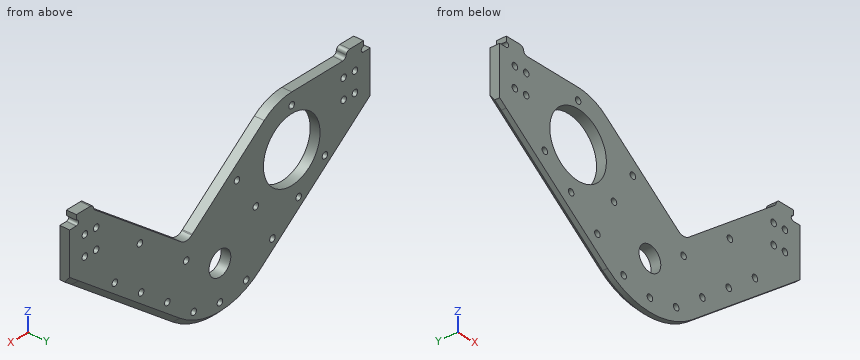
from build123d import *

# Parameters (mm, degrees)
SKETCH3_R                          = 17.8
SKETCH3_R_2                        = 7.9375
BOSS_EXTRUDE1_DEPTH                = 6.35
SKETCH7_R                          = 20.6375
CUT_EXTRUDE1_DEPTH                 = 7.35
SKETCH8_W                          = 4.7498
SKETCH8_H                          = 41.275
BOSS_EXTRUDE4_DEPTH                = 6.35
SKETCH10_R                         = 2.0193
SPACER_HOLES_DEPTH                 = 7.35
SPACER_HOLE_PATTERN_COUNT          = 5
SPACER_HOLE_PATTERN_PITCH          = 24.13
SPACER_HOLE_MIRROR_COPY_1_SKETCH_R = 2.0193
SPACER_HOLE_MIRROR_COPY_1_DEPTH    = 7.35
SPACER_HOLE_MIRROR_COPY_2_SKETCH_R = 2.0193
SPACER_HOLE_MIRROR_COPY_2_DEPTH    = 7.35
SPACER_HOLE_MIRROR_COPY_3_SKETCH_R = 2.0193
SPACER_HOLE_MIRROR_COPY_3_DEPTH    = 7.35
SPACER_HOLE_MIRROR_COPY_4_SKETCH_R = 2.0193
SPACER_HOLE_MIRROR_COPY_4_DEPTH    = 7.35
SPACER_HOLE_MIRROR_COPY_5_SKETCH_R = 2.0193
SPACER_HOLE_MIRROR_COPY_5_DEPTH    = 7.35
SKETCH16_R                         = 2.0193
CUSTOM_NUTSTRIP_HOLES_DEPTH        = 7.35
SKETCH36_R                         = 2.0193
AUX_SPACER_HOLES_DEPTH             = 7.35
SKETCH58_R                         = 2.0193
CUT_EXTRUDE30_DEPTH                = 7.35
SKETCH84_R                         = 2.0193
CUT_EXTRUDE40_DEPTH                = 7.35
CUT_EXTRUDE34_DEPTH                = 7.35
SKETCH105_W                        = 4.8768
SKETCH105_H                        = 6.477
CUT_EXTRUDE54_DEPTH                = 7.35
SKETCH106_R                        = 1.651
CUT_EXTRUDE55_DEPTH                = 7.35
CHAMFER5_SIZE                      = 3.175
FILLET21_R                         = 6.35
FILLET22_R                         = 2.54
FILLET23_R                         = 2.54


with BuildPart() as part:
    # Sketch3 → Boss-Extrude1 (new body)
    with BuildSketch(Plane(origin=(0, 25.4, 0), x_dir=(1, 0, 0), z_dir=(0, 1, 0))):
        with BuildLine():
            Line((-104.775, -36.374686106), (-30.925080594, 20.292350114))
            Line((-30.925080594, 20.292350114), (0, 44.021999059))
            Line((0, 44.021999059), (30.925080594, 20.292350114))
            Line((30.925080594, 20.292350114), (104.775, -36.374686106))
            Line((104.775, -36.374686106), (104.775, -77.649686106))
            Line((104.775, -77.649686106), (92.075, -77.649686106))
            Line((92.075, -77.649686106), (92.075, -74.653632333))
            Line((92.075, -74.653632333), (24.142327736, -22.527059539))
            ThreePointArc((24.142327736, -22.527059539), (22.197769032, -24.445438225), (20.101302386, -26.196527296))
            Line((20.101302386, -26.196527296), (-32.251449857, -66.368206988))
            ThreePointArc((-32.251449857, -66.368206988), (-41.738821099, -71.439312567), (-52.352752243, -73.191679691))
            Line((-52.352752243, -73.191679691), (-92.075, -73.191679691))
            Line((-92.075, -73.191679691), (-92.075, -77.649686106))
            Line((-92.075, -77.649686106), (-104.775, -77.649686106))
            Line((-104.775, -77.649686106), (-104.775, -36.374686106))
        make_face()
        with Locations((-52.352752243, -40.171679691)):
            Circle(SKETCH3_R, mode=Mode.SUBTRACT)
        Circle(SKETCH3_R_2, mode=Mode.SUBTRACT)
    extrude(amount=-BOSS_EXTRUDE1_DEPTH)

    # Sketch7 → Cut-Extrude1 (cut, through all)
    with BuildSketch(Plane(origin=(0, 25.4, 0), x_dir=(1, 0, 0), z_dir=(0, 1, 0))):
        with Locations((-52.352752243, -40.171679691)):
            Circle(SKETCH7_R)
    extrude(amount=-CUT_EXTRUDE1_DEPTH, mode=Mode.SUBTRACT)

    # Sketch8 → Boss-Extrude4 (add, through all)
    with BuildSketch(Plane(origin=(0, 25.4, 0), x_dir=(1, 0, 0), z_dir=(0, 1, 0))):
        with Locations((-107.1499, -57.012186106)):
            Rectangle(SKETCH8_W, SKETCH8_H)
        with Locations((107.1499, -57.012186106)):
            Rectangle(SKETCH8_W, SKETCH8_H)
    extrude(amount=-BOSS_EXTRUDE4_DEPTH)

    # Sketch10 → Spacer Holes (cut, through all)
    with BuildSketch(Plane(origin=(0, 25.4, 0), x_dir=(1, 0, 0), z_dir=(0, 1, 0))):
        with Locations((0, 33.456719285)):
            Circle(SKETCH10_R)
    spacer_holes = extrude(amount=-SPACER_HOLES_DEPTH, mode=Mode.SUBTRACT)

    # Spacer Hole Pattern: Spacer Holes ×5
    with Locations(*[Vector(-0.79335334, 0, 0.608761429) * (i * SPACER_HOLE_PATTERN_PITCH) for i in range(1, SPACER_HOLE_PATTERN_COUNT)]):
        add(spacer_holes, mode=Mode.SUBTRACT)

    # Spacer Hole Mirror copy 1 sketch → Spacer Hole Mirror copy 1 (cut, through all)
    with BuildSketch(Plane(origin=(19.143616101, 25.4, 14.689413282), x_dir=(-1, 0, 0), z_dir=(0, 1, 0))):
        with Locations((0, -33.456719285)):
            Circle(SPACER_HOLE_MIRROR_COPY_1_SKETCH_R)
    extrude(amount=-SPACER_HOLE_MIRROR_COPY_1_DEPTH, mode=Mode.SUBTRACT)

    # Spacer Hole Mirror copy 2 sketch → Spacer Hole Mirror copy 2 (cut, through all)
    with BuildSketch(Plane(origin=(38.287232202, 25.4, 29.378826564), x_dir=(-1, 0, 0), z_dir=(0, 1, 0))):
        with Locations((0, -33.456719285)):
            Circle(SPACER_HOLE_MIRROR_COPY_2_SKETCH_R)
    extrude(amount=-SPACER_HOLE_MIRROR_COPY_2_DEPTH, mode=Mode.SUBTRACT)

    # Spacer Hole Mirror copy 3 sketch → Spacer Hole Mirror copy 3 (cut, through all)
    with BuildSketch(Plane(origin=(57.430848304, 25.4, 44.068239846), x_dir=(-1, 0, 0), z_dir=(0, 1, 0))):
        with Locations((0, -33.456719285)):
            Circle(SPACER_HOLE_MIRROR_COPY_3_SKETCH_R)
    extrude(amount=-SPACER_HOLE_MIRROR_COPY_3_DEPTH, mode=Mode.SUBTRACT)

    # Spacer Hole Mirror copy 4 sketch → Spacer Hole Mirror copy 4 (cut, through all)
    with BuildSketch(Plane(origin=(76.574464405, 25.4, 58.757653128), x_dir=(-1, 0, 0), z_dir=(0, 1, 0))):
        with Locations((0, -33.456719285)):
            Circle(SPACER_HOLE_MIRROR_COPY_4_SKETCH_R)
    extrude(amount=-SPACER_HOLE_MIRROR_COPY_4_DEPTH, mode=Mode.SUBTRACT)

    # Spacer Hole Mirror copy 5 sketch → Spacer Hole Mirror copy 5 (cut, through all)
    with BuildSketch(Plane(origin=(0, 25.4, 0), x_dir=(-1, 0, 0), z_dir=(0, 1, 0))):
        with Locations((0, -33.456719285)):
            Circle(SPACER_HOLE_MIRROR_COPY_5_SKETCH_R)
    extrude(amount=-SPACER_HOLE_MIRROR_COPY_5_DEPTH, mode=Mode.SUBTRACT)

    # Sketch16 → Custom Nutstrip Holes (cut, through all)
    with BuildSketch(Plane(origin=(0, 25.4, 0), x_dir=(1, 0, 0), z_dir=(0, 1, 0))):
        with Locations((-98.425, -50.662186106)):
            Circle(SKETCH16_R)
        with Locations((-98.425, -63.362186106)):
            Circle(SKETCH16_R)
        with Locations((98.425, -63.362186106)):
            Circle(SKETCH16_R)
        with Locations((98.425, -50.662186106)):
            Circle(SKETCH16_R)
    extrude(amount=-CUSTOM_NUTSTRIP_HOLES_DEPTH, mode=Mode.SUBTRACT)

    # Sketch36 → Aux Spacer Holes (cut, through all)
    with BuildSketch(Plane(origin=(0, 25.4, 0), x_dir=(1, 0, 0), z_dir=(0, 1, 0))):
        with Locations((-52.352752243, -65.571679691)):
            Circle(SKETCH36_R)
        with Locations((58.293943402, -39.127716128)):
            Circle(SKETCH36_R)
        with Locations((24.512886804, -13.206599718)):
            Circle(SKETCH36_R)
        with Locations((-12.439980265, -41.561531903)):
            Circle(SKETCH36_R)
        with Locations((-26.176376122, -20.085839846)):
            Circle(SKETCH36_R)
    extrude(amount=-AUX_SPACER_HOLES_DEPTH, mode=Mode.SUBTRACT)

    # Sketch58 → Cut-Extrude30 (cut, through all)
    with BuildSketch(Plane(origin=(0, 25.4, 0), x_dir=(1, 0, 0), z_dir=(0, 1, 0))):
        with Locations((0, 22.408000428)):
            Circle(SKETCH58_R)
        with BuildLine():
            Line((-30.925080594, 20.292350114), (0, 44.021999059))
            Line((0, 44.021999059), (30.925080594, 20.292350114))
            ThreePointArc((30.925080594, 20.292350114), (0, 30.790000428), (-30.925080594, 20.292350114))
        make_face()
    extrude(amount=-CUT_EXTRUDE30_DEPTH, mode=Mode.SUBTRACT)

    # Sketch84 → Cut-Extrude40 (cut, through all)
    with BuildSketch(Plane(origin=(0, 25.4, 0), x_dir=(1, 0, 0), z_dir=(0, 1, 0))):
        with Locations((90.17, -50.662186106)):
            Circle(SKETCH84_R)
        with Locations((90.17, -63.362186106)):
            Circle(SKETCH84_R)
        with Locations((-90.17, -50.662186106)):
            Circle(SKETCH84_R)
        with Locations((-90.17, -63.362186106)):
            Circle(SKETCH84_R)
    extrude(amount=-CUT_EXTRUDE40_DEPTH, mode=Mode.SUBTRACT)

    # Sketch75 → Cut-Extrude34 (cut, through all)
    with BuildSketch(Plane(origin=(0, 25.4, 0), x_dir=(1, 0, 0), z_dir=(0, 1, 0))):
        Polygon((-104.775, -36.374686106), (-109.5248, -40.019335834), (-109.5248, -36.374686106), align=None)
        Polygon((104.775, -36.374686106), (109.5248, -40.019335834), (109.5248, -36.374686106), align=None)
    extrude(amount=-CUT_EXTRUDE34_DEPTH, mode=Mode.SUBTRACT)

    # Sketch105 → Cut-Extrude54 (cut, through all)
    with BuildSketch(Plane(origin=(0, 25.4, 0), x_dir=(1, 0, 0), z_dir=(0, 1, 0))):
        with Locations((-107.0864, -74.411186106)):
            Rectangle(SKETCH105_W, SKETCH105_H)
        with Locations((107.0864, -74.411186106)):
            Rectangle(SKETCH105_W, SKETCH105_H)
    extrude(amount=-CUT_EXTRUDE54_DEPTH, mode=Mode.SUBTRACT)

    # Sketch106 → Cut-Extrude55 (cut, through all)
    with BuildSketch(Plane(origin=(0, 25.4, 0), x_dir=(1, 0, 0), z_dir=(0, 1, 0))):
        with Locations((-104.648, -72.823686106)):
            Circle(SKETCH106_R)
        with Locations((104.648, -72.823686106)):
            Circle(SKETCH106_R)
    extrude(amount=-CUT_EXTRUDE55_DEPTH, mode=Mode.SUBTRACT)

    # Chamfer5
    chamfer5_edges = [part.edges().sort_by_distance(p)[0] for p in [
        (70.224940297, 25.4, 9.86349286),
        (-70.224940297, 25.4, 9.86349286),
        (0, 25.4, -30.790000428),
    ]]
    chamfer(chamfer5_edges, length=CHAMFER5_SIZE)

    # Fillet21
    fillet21_edges = [part.edges().sort_by_distance(p)[0] for p in [
        (24.142327736, 22.225, 22.527059539),
    ]]
    fillet(fillet21_edges, radius=FILLET21_R)

    # Fillet22
    fillet22_edges = [part.edges().sort_by_distance(p)[0] for p in [
        (-92.075, 22.225, 73.191679691),
        (92.075, 22.225, 74.653632333),
    ]]
    fillet(fillet22_edges, radius=FILLET22_R)

    # Fillet23
    fillet23_edges = [part.edges().sort_by_distance(p)[0] for p in [
        (92.075, 22.225, 77.649686106),
        (-92.075, 22.225, 77.649686106),
    ]]
    fillet(fillet23_edges, radius=FILLET23_R)


solid = part.part
Check sheet for the modelled part. Datum: model origin and axes. Units: mm. Coordinates: 2 decimals unless noted, no trailing zeros. Loops run counter-clockwise (first coordinate to the right, second up) from the corner with the lowest first, then second, coordinate; pieces in that order, holes last. Notation, with made-up numbers: (7, 12) -> (48, 12) arc R22 cw to (48, 32) -> close; hole circle Ø10 at (-15, 88). An arc over 180 degrees is marked (long way). Answer in a Markdown table with one row per item.
1. Sectioned sample at D-D, the plane z = -11. Record the boundary of the cut face in (x, y) (3 decimals).
Check values:
| item | result |
|---|---|
| outline | (-43.035, 19.05) -> (43.035, 19.05) -> (43.035, 22.225) -> (37.82, 25.4) -> (-37.82, 25.4) -> (-43.035, 22.225) -> close |
2. Sectioned sample at B-B, the plane x = -46.5. Record the boundary of the cut face in (y, z) (3 decimals), then the cut area to 3 significant figures.
Check values:
| item | result |
|---|---|
| outline | (19.05, -8.341) -> (22.225, -8.341) -> (25.4, -4.339) -> (25.4, 20.381) -> (19.05, 20.381) -> close; (19.05, 59.962) -> (25.4, 59.962) -> (25.4, 72.669) -> (19.05, 72.669) -> close |
| area | 257 mm2 |
3. Sectioned sample at A-A, the plane x = 0. Give the number of separate pieces and of enclosed holes in the cut face, then the cut area to 3 significant figures.
Check values:
| item | result |
|---|---|
| separate pieces | 3 |
| enclosed holes | 0 |
| area | 328 mm2 |
4. Go/stop test with flat-tipped pins: pin 1 (3 mm diameter, centred on x = -52.35, z = 65.57, fed in from +Y); pin 2 (1.5 mm diameter, centred on x = -107, y = 21.5, fed in from +Z); pin 3 (3.5 mm diameter, centred on y = 20.5, z = 75.5, fed in from +X); pin 4 (2 mm diameter, centred on y = 24, z = 36, fed in from -X). Record where each tip stops, or that it passes through.
Check values:
| item | result |
|---|---|
| pin 1 | passes through |
| pin 2 | stops at z = 71.17 |
| pin 3 | stops at x = 104.65 |
| pin 4 | stops at x = -103.47 |
5. Material ranges on line 1 along X through (y, z) = (21.5, 44); line 2 along Z through (x, y) = (-51.5, 19.75); line 3 along X through (y, z) = (22.25, 21.5), recorded low to high. Write a range as [from, to].
Check values:
| item | result |
|---|---|
| line 1 | x = [-109.52, -72.63], [-32.07, -3.1], [52.13, 109.52] |
| line 2 | z = [-4.5, 19.55], [60.79, 63.74], [67.4, 73.18] |
| line 3 | x = [-85.35, -61.14], [-43.56, -27.62], [-24.73, 85.35] |
